Source: CAD feature listing. Evaluate the final solid. Frame: model axes, mm. A direction names the side the tool comes from. Coordinates: 2 decimals unless noted, no trailing zeros. Order: outer loops, then holes, each group sorted by start corner. A loop starts at its lowest first (then second) coordinate and runs counter-clockwise, first axis right, second up.
Autodesk Inventor part; units mm, degrees
ref_plane "Work Plane1" through (-60, -55, 0) normal (0, -1, 0) x (1, 0, 0)
ref_plane "YZ Plane" through (0, 0, 0) normal (1, 0, 0) x (0, 1, 0)
ref_plane "XZ Plane" through (0, 0, 0) normal (0, 1, 0) x (-1, 0, 0)
sketch "Sketch1" plane through (0, 0, 0) normal (0, 0, 1) x (1, 0, 0)
  circle A0 centre (0, 0) radius 47.525
  arc A1 (60, 0) -> (-60, 0) centre (0, 0) ccw
  line L0 (-60, 0) -> (-60, -70)
  line L1 (-60, -70) -> (60, -70)
  line L2 (60, -70) -> (60, 0)
  dimension "d0" = 95.05
  dimension "d2" = 70
  dimension "d43" = 60
extrude "Extrusion1" add sketch "Sketch1" along normal blind 32.5
sketch "Sketch2" plane through (0, 0, 0) normal (0, 0, -1) x (-1, 0, 0)
  circle A0 centre (0, 0) radius 47.525
  circle A1 centre (0, 0) radius 45.525
  dimension "d5" = 2
extrude "Extrusion2" add sketch "Sketch2" against normal blind 1
sketch "Sketch3" plane through (0, 0, 32.5) normal (0, 0, 1) x (1, 0, 0)
  arc A0 (60, 0) -> (-60, 0) centre (0, 0) ccw construction
  line L0 (0, 0) -> (0, 55) construction
  circle A1 centre (0, 55) radius 2.6
  circle A2 centre (-52.3081, 16.9959) radius 2.6
  circle A3 centre (-32.3282, -44.4959) radius 2.6
  circle A4 centre (32.3282, -44.4959) radius 2.6
  circle A5 centre (52.3081, 16.9959) radius 2.6
  dimension "d8" = 5.2
  dimension "d9" = 55
  dimension "d12" = 360
extrude "Extrusion3" cut sketch "Sketch3" against normal through all
sketch "Sketch7" plane through (-60, -70, 0) normal (-1, 0, 0) x (0, 0, 1)
  line L0 (0, 0) -> (32.5, 0)
  line L1 (0, 0) -> (-30, 0)
  line L2 (-30, 0) -> (-30, 5)
  line L3 (0, 70) -> (0, 0)
  line L4 (-30, 5) -> (0, 35)
  line L5 (0, 0) -> (0, 35)
  dimension "d32" = 30
  dimension "d33" = 5
  dimension "d34" = 135
extrude "Extrusion7" add sketch "Sketch7" against normal blind 15
mirror "Mirror1" about plane through (0, 0, 0) normal (1, 0, 0) of "Extrusion7"
sketch "Sketch5" plane through (-60, -70, 0) normal (0, -1, 0) x (1, 0, 0)
  circle A0 centre (7.5, 25) radius 2.75
  circle A1 centre (112.5, 25) radius 2.75
  circle A2 centre (86.25, 7.5) radius 2.75
  circle A3 centre (33.75, 7.5) radius 2.75
  circle A4 centre (60, 25) radius 2.75
  line L0 (7.5, 25) -> (60, 25) construction
  line L1 (60, 25) -> (112.5, 25) construction
  line L2 (86.25, 7.5) -> (33.75, 7.5) construction
  line L3 (60, 25) -> (60, 7.5) construction
  line L4 (60, 7.5) -> (60, 0) construction
  line L5 (0, 0) -> (120, 0) construction
  line L6 (0, 32.5) -> (120, 32.5) construction
  line L7 (0, 0) -> (0, 32.5) construction
  line L8 (33.75, 25) -> (33.75, 7.5) construction
  line L9 (0, -30) -> (15, -30) construction
  line L10 (7.5, -30) -> (7.5, -20) construction
  line L11 (120, -30) -> (105, -30) construction
  line L12 (112.5, -30) -> (112.5, -20) construction
  line L13 (112.5, -20) -> (7.5, -20) construction
  circle A5 centre (7.5, -20) radius 2.75
  circle A6 centre (112.5, -20) radius 2.75
  line L14 (112.5, -20) -> (112.5, 25) construction
  line L15 (120, -30) -> (120, 32.5)
  dimension "d16" = 5.5
  dimension "d17" = 7.5
  dimension "d18" = 7.5
  dimension "d37" = 10
  dimension "d39" = 17.5
  dimension "d45" = 52.5
  dimension "d46" = 45
  dimension "d47" = 7.5
extrude "Extrusion4" cut sketch "Sketch5" against normal blind 18
ref_plane "Work Plane1" through (-60, -55, 0) normal (0, -1, 0) x (1, 0, 0)
sketch "Sketch6" plane through (-60, -55, 0) normal (0, -1, 0) x (1, 0, 0)
  circle A0 centre (112.5, 25) radius 2.75
  circle A1 centre (60, 25) radius 2.75
  circle A2 centre (33.75, 7.5) radius 2.75
  line L0 (112.5, 29.7343) -> (116.6, 27.3671) construction
  line L1 (116.6, 27.3671) -> (116.6, 22.6329)
  line L2 (116.6, 22.6329) -> (112.5, 20.2657)
  line L3 (112.5, 20.2657) -> (108.4, 22.6329)
  line L4 (108.4, 22.6329) -> (108.4, 27.3671)
  line L5 (108.4, 27.3671) -> (112.5, 29.7343) construction
  line L6 (60, 29.7343) -> (64.1, 27.3671)
  line L7 (64.1, 27.3671) -> (64.1, 22.6329)
  line L8 (64.1, 22.6329) -> (60, 20.2657)
  line L9 (60, 20.2657) -> (55.9, 22.6329)
  line L10 (55.9, 22.6329) -> (55.9, 27.3671)
  line L11 (55.9, 27.3671) -> (60, 29.7343)
  circle A3 centre (33.75, 7.5) radius 2.75
  line L12 (33.75, 2.7657) -> (29.65, 5.1329) construction
  line L13 (29.65, 5.1329) -> (29.65, 9.8671)
  line L14 (29.65, 9.8671) -> (33.75, 12.2343)
  line L15 (33.75, 12.2343) -> (37.85, 9.8671)
  line L16 (37.85, 9.8671) -> (37.85, 5.1329)
  line L17 (37.85, 5.1329) -> (33.75, 2.7657) construction
  circle A4 centre (86.25, 7.5) radius 2.75
  line L18 (86.25, 2.7657) -> (82.15, 5.1329) construction
  line L19 (82.15, 5.1329) -> (82.15, 9.8671)
  line L20 (82.15, 9.8671) -> (86.25, 12.2343)
  line L21 (86.25, 12.2343) -> (90.35, 9.8671)
  line L22 (90.35, 9.8671) -> (90.35, 5.1329)
  line L23 (90.35, 5.1329) -> (86.25, 2.7657) construction
  circle A5 centre (7.5, 25) radius 2.75
  line L24 (7.5, 20.2657) -> (3.4, 22.6329)
  line L25 (3.4, 22.6329) -> (3.4, 27.3671)
  line L26 (3.4, 27.3671) -> (7.5, 29.7343) construction
  line L27 (7.5, 29.7343) -> (11.6, 27.3671) construction
  line L28 (11.6, 27.3671) -> (11.6, 22.6329)
  line L29 (11.6, 22.6329) -> (7.5, 20.2657)
  line L30 (116.6, 27.3671) -> (116.6, 35.5137)
  line L31 (116.6, 35.5137) -> (108.4, 35.5137)
  line L32 (108.4, 35.5137) -> (108.4, 27.3671)
  line L33 (90.35, 5.1329) -> (90.35, -3.3085)
  line L34 (90.35, -3.3085) -> (82.15, -3.3085)
  line L35 (82.15, -3.3085) -> (82.15, 5.1329)
  line L36 (37.85, 5.1329) -> (37.85, -3.965)
  line L37 (37.85, -3.965) -> (29.65, -3.965)
  line L38 (29.65, -3.965) -> (29.65, 5.1329)
  line L39 (12.475, 1) -> (107.525, 1)
  line L40 (11.6, 27.3671) -> (11.6, 33.5607)
  line L41 (11.6, 33.5607) -> (3.4, 33.5607)
  line L42 (3.4, 33.5607) -> (3.4, 27.3671)
  circle A6 centre (112.5, -20) radius 2.75
  circle A7 centre (112.5, -20) radius 2.75
  circle A8 centre (7.5, -20) radius 2.75
  line L43 (112.5, -24.7343) -> (108.4, -22.3671)
  line L44 (108.4, -22.3671) -> (108.4, -17.6329)
  line L45 (108.4, -17.6329) -> (112.5, -15.2657)
  line L46 (112.5, -15.2657) -> (116.6, -17.6329)
  line L47 (116.6, -17.6329) -> (116.6, -22.3671)
  line L48 (116.6, -22.3671) -> (112.5, -24.7343)
  line L49 (7.5, -24.7343) -> (3.4, -22.3671)
  line L50 (3.4, -22.3671) -> (3.4, -17.6329)
  line L51 (3.4, -17.6329) -> (7.5, -15.2657)
  line L52 (7.5, -15.2657) -> (11.6, -17.6329)
  line L53 (11.6, -17.6329) -> (11.6, -22.3671)
  line L54 (11.6, -22.3671) -> (7.5, -24.7343)
  point P0 (60, 0)
  point P1 (60, 25)
  point P2 (33.75, 7.5)
  point P3 (7.5, 25)
  point P4 (37.85, 1)
  point P5 (29.65, 1)
  point P6 (90.35, 1)
  point P7 (82.15, 1)
  point P8 (7.5, -20)
  dimension "d23" = 8.2
extrude "Extrusion5" cut sketch "Sketch6" along normal blind 4.5 contours A1 | L1 L2 L3 L4 L32 L31 L30 | L6 L7 L8 L9 L10 L11 | L35 L19 L20 L21 L22 L33 L39 | L39 L33 L34 L35 | L13 L14 L15 L16 L36 L39 L38 | L39 L36 L37 L38 | L24 L25 L42 L41 L40 L28 L29 | L43 L44 L45 L46 L47 L48 | L49 L50 L51 L52 L53 L54
extrude "Extrusion6" cut sketch "Sketch6" against normal blind 20.75 contours A1 | L6 L7 L8 L9 L10 L11 | L43 L44 L45 L46 L47 L48 | L49 L50 L51 L52 L53 L54
fillet "Fillet1" radius 2 1 edges at (-47.525, 0, 32.5)
chamfer "Chamfer1" distance 2 angle 45 10 edges at (0, 60, 32.5) (-60, -35, 32.5) (60, -35, 32.5) (0, 60, 0) (-60, -17.5, 0) (60, -17.5, 0) (-60, -50, -15) (-45, -50, -15) (45, -50, -15) (60, -50, -15)
fillet "Fillet2" radius 5 4 edges at (-45, -53.9142, 0) (45, -53.9142, 0) (52.5, -35, 0) (-52.5, -35, 0)
chamfer "Chamfer2" distance 2 angle 45 1 edges at (-47.525, 0, 1)
sketch "Sketch9" plane through (0, 0, 32.5) normal (0, 0, 1) x (1, 0, 0)
  circle A0 centre (0, 0) radius 47.525
  circle A1 centre (0, 0) radius 47.525
extrude "Extrusion8" cut sketch "Sketch9" against normal through all
sketch "Sketch10" plane through (0, 0, 32.5) normal (0, 0, 1) x (1, 0, 0)
  circle A0 centre (-32.3282, -44.4959) radius 2.6
  circle A1 centre (-52.3081, 16.9959) radius 2.6
  circle A2 centre (0, 55) radius 2.6
  circle A3 centre (52.3081, 16.9959) radius 2.6
  circle A4 centre (32.3282, -44.4959) radius 2.6
  point P0 (0, 0)
extrude "Extrusion9" add sketch "Sketch10" against normal up to surface (32.5 mm away)
sketch "Sketch11" plane through (0, 0, 32.5) normal (0, 0, 1) x (1, 0, 0)
  circle A0 centre (0, 0) radius 49.525
extrude "Extrusion10" add sketch "Sketch11" against normal blind 3
equation "\"d17\" = d47"
equation "\"d18\" = d47"
properties part number "J1_idlebracket"
Q1. Set-up query: faces 1 (the cylindrical face through (-43, -56, -1)), 2 (the flat face through (-4.1, -54, 25)), 3 (the flat face through (-22.15, -57, 5)), 4 (the flat face through (60, -42, 14)), 5 (the flat face through (52, -52, 25)). Return all of +Z, -Z, +X, -X, +Y, -Y with unobstructed straight access to the full face (end or side cutting, diameter ignored); none if empty.
Solutions:
face 1: -Z, +Y, -Y
face 2: none
face 3: -Z
face 4: +Z, -Z, +X, +Y, -Y
face 5: -Y
Q2. Section query B-B on y = -16. Output: boundary loops of the cut face in (x, z), plus the area to 3 significant figures.
Solutions:
outline: (-60, 2) - (-58, 0) - (-44.75, 0) - (-44.75, 29.5) - (44.75, 29.5) - (44.75, 0) - (58, 0) - (60, 2) - (60, 30.5) - (58, 32.5) - (-58, 32.5) - (-60, 30.5) - close
area: 1,250 mm2
Q3. Section query A-A on z = -12. Output: boundary loops of the cut face in (x, y), plus the area to 3 significant figures.
Solutions:
outline: (-60, -70) - (-45, -70) - (-45, -49.83) - (-47, -47) - (-58, -47) - (-60, -49.83) - close; (45, -70) - (60, -70) - (60, -49.83) - (58, -47) - (47, -47) - (45, -49.83) - close
area: 679 mm2
Q4. Pin query (flat end, axial travel): P1, Ø1.6, axis at x = -54, z = 26, coming from the -Y side; P2, Ø1.5, axis at y = 33, z = 8.5, coming from the -X side; P3, Ø5, axis at x = 52.5, z = 25, coming from the +Y side. Return the tip coordinate at first contact, or that it passes through.
Solutions:
P1: stops at y = -52
P2: stops at x = -50.6
P3: stops at y = 33.17
Q5. Material intervals for line 1 along Z through (x, y) = (52.5, -65.25); line 2 along X through (y, z) = (0, 14) (3 decimals); line 3 along Z through (x, y) = (52.5, -53.1), sorted ascending.
Solutions:
line 1: z = -30 to -22.75, -17.25 to 22.25, 27.75 to 32.5
line 2: x = -60 to -47.525, 47.525 to 60
line 3: z = -15.27 to 22.25, 27.75 to 32.5
Q6. Section query D-D on z = -3. Output: boundary loops of the cut face in (x, y).
Solutions:
outline: (-60, -70) - (-44.58, -70) - (-44.58, -41.42) - (-47, -38) - (-58, -38) - (-60, -40.83) - close; (44.58, -70) - (60, -70) - (60, -40.83) - (58, -38) - (47, -38) - (44.58, -41.42) - close
Q7. Section query C-C on z = 18. Output: boundary loops of the cut face in (x, y) (3 decimals).
Solutions:
outline: (-60, -70) - (60, -70) - (60, 0) arc R60 ccw to (-60, 0) - close; hole circle Ø95.05 at (0, 0)
Q8. Pull-direction query (Z, two-part tool) for faces 6 (the flat face through (48.4, -57, 27)), 7 (the cylindrical face through (44, -56, -2)), 8 (the cylindrical face through (-55.247, -53.521, 25.121)), 9 (the cylindrical face through (23.5, -64.8, 7.6)); classes: pulls with the +Z half, pulls with the -Z half, needs draft (parallel to the pull), parting line crosses it, or undercut.
Solutions:
face 6: needs draft
face 7: pulls with the -Z half
face 8: undercut
face 9: undercut
